```python
from build123d import *

# Parameters (mm, degrees)
SKETCH_1_R              = 8
EXTRUDE_1_DEPTH         = 3
HOLE_WIZARD_M1_21_D     = 1.4
HOLE_WIZARD_M1_21_DEPTH = 9.579397567
HOLE_WIZARD_M1_21_TIP   = 0.420602433
SKETCH_1_3_R            = 18
EXTRUDE_2_DEPTH         = 2
SKETCH_2_W              = 16
SKETCH_2_H              = 7
EXTRUDE_3_DEPTH         = 27
FILLET_1_R              = 6
FILLET_3_R              = 1.5
HOLE_WIZARD_M21_D       = 2.4
HOLE_WIZARD_M21_DEPTH   = 9.278967257
HOLE_WIZARD_M21_TIP     = 0.721032743
HOLE_WIZARD_M1_22_D     = 1.4
HOLE_WIZARD_M1_22_DEPTH = 9.579397567
HOLE_WIZARD_M1_22_TIP   = 0.420602433
FILLET_4_R              = 2


with BuildPart() as part:
    # Sketch 1 → Extrude 1 (new body)
    with BuildSketch(Plane.XY):
        with BuildLine():
            Line((0, 0), (40, 0))
            ThreePointArc((40, 0), (49.772170092, 28), (40, 56))
            Line((40, 56), (0, 56))
            Line((0, 56), (0, 0))
        make_face()
        with Locations((20, 28)):
            Circle(SKETCH_1_R, mode=Mode.SUBTRACT)
    extrude(amount=-EXTRUDE_1_DEPTH)

    # Hole Wizard M1.21
    with Locations(Plane.XY):
        with Locations((20, 41), (31.258330249, 34.5), (31.258330249, 21.5), (20, 15), (8.741669751, 21.5), (8.741669751, 34.5)):
            Hole(HOLE_WIZARD_M1_21_D / 2, depth=HOLE_WIZARD_M1_21_DEPTH)
            with Locations((0, 0, -(HOLE_WIZARD_M1_21_DEPTH + HOLE_WIZARD_M1_21_TIP / 2))):  # 118° drill point
                Cone(0, HOLE_WIZARD_M1_21_D / 2, HOLE_WIZARD_M1_21_TIP, mode=Mode.SUBTRACT)

    # Sketch 1_3 → Extrude 2 (add)
    with BuildSketch(Plane.XY):
        with BuildLine():
            Line((0, 0), (40, 0))
            ThreePointArc((40, 0), (49.772170092, 28), (40, 56))
            Line((40, 56), (0, 56))
            Line((0, 56), (0, 0))
        make_face()
        with Locations((20, 28)):
            Circle(SKETCH_1_3_R, mode=Mode.SUBTRACT)
    extrude(amount=EXTRUDE_2_DEPTH)

    # Sketch 2 → Extrude 3 (add)
    with BuildSketch(Plane.XY.offset(2)):
        with BuildLine():
            Line((40, 0), (12, 0))
            Line((12, 0), (12, 7))
            Line((12, 7), (40, 7))
            Line((40, 7), (40, 49))
            Line((40, 49), (38, 49))
            Line((38, 49), (38, 56))
            Line((38, 56), (40, 56))
            ThreePointArc((40, 56), (49.772170092, 28), (40, 0))
        make_face()
        with Locations((20, 52.5)):
            Rectangle(SKETCH_2_W, SKETCH_2_H)
    extrude(amount=EXTRUDE_3_DEPTH)

    # Fillet 1
    fillet_1_edges = [part.edges().sort_by_distance(p)[0] for p in [
        (40, 56, 13),
        (40, 0, 13),
        (0, 0, -0.5),
        (0, 56, -0.5),
    ]]
    fillet(fillet_1_edges, radius=FILLET_1_R)

    # Fillet 3
    fillet_3_edges = [part.edges().sort_by_distance(p)[0] for p in [
        (12, 7, 15.5),
        (12, 0, 15.5),
        (12, 56, 15.5),
        (12, 49, 15.5),
        (28, 49, 15.5),
        (28, 56, 15.5),
    ]]
    fillet(fillet_3_edges, radius=FILLET_3_R)

    # Hole Wizard M21
    with Locations(Plane.XY.offset(29)):
        with Locations((44, 38), (44, 18)):
            Hole(HOLE_WIZARD_M21_D / 2, depth=HOLE_WIZARD_M21_DEPTH)
            with Locations((0, 0, -(HOLE_WIZARD_M21_DEPTH + HOLE_WIZARD_M21_TIP / 2))):  # 118° drill point
                Cone(0, HOLE_WIZARD_M21_D / 2, HOLE_WIZARD_M21_TIP, mode=Mode.SUBTRACT)

    # Hole Wizard M1.22
    with Locations(Plane.ZY.offset(-12)):
        with Locations((20, 52.240238149), (11, 52.240238149), (20, 3.759761857), (11, 3.759761857)):
            Hole(HOLE_WIZARD_M1_22_D / 2, depth=HOLE_WIZARD_M1_22_DEPTH)
            with Locations((0, 0, -(HOLE_WIZARD_M1_22_DEPTH + HOLE_WIZARD_M1_22_TIP / 2))):  # 118° drill point
                Cone(0, HOLE_WIZARD_M1_22_D / 2, HOLE_WIZARD_M1_22_TIP, mode=Mode.SUBTRACT)

    # Fillet 4
    fillet_4_edges = [part.edges().sort_by_distance(p)[0] for p in [
        (49.772170092, 28, -3),
        (21.487327234, 56, -3),
        (21.487327234, 0, -3),
        (0, 28, -3),
        (1.757359313, 54.242640687, -3),
        (1.757359313, 1.757359313, -3),
        (39.775753154, 0.693980197, -3),
        (39.775753154, 55.306019803, -3),
    ]]
    fillet(fillet_4_edges, radius=FILLET_4_R)


solid = part.part
```
Geometry check sheet. Reference: the model listing, model coordinates, mm. A direction names the side the tool comes from. Round coordinates to 2 decimals unless told otherwise and drop trailing zeros. Order: outer loops, then holes, each group sorted by start corner. A loop starts at its lowest first (then second) coordinate and runs counter-clockwise, first axis right, second up. Notation, with made-up numbers: (29.25, 72.25) - (62.25, 72.25) arc R36 cw to (62.25, 110.25) - close; hole circle Ø11 at (10, 17). An arc over 180 degrees is marked (long way). Use a Markdown table: item, result. Add a question column.
1) Set-up check for faces 5 (the cylindrical face through (42.89, 17.54, 24.3)), 6 (the cylindrical face through (21.27, 55.4, -2.43)), 7 (the flat face through (39, 49, 15)), 8 (the flat face through (0, 28, 0)), 9 (the flat face through (12, 3, 15)): record each of +Z, -Z, +X, -X, +Y, -Y from which the full face is reachable in a straight line by a thin tool's end or side.
2) Section check A-A (z = 21.5). Record the cut outline in (x, y), then the cut area to 3 significant figures.
3) Section check B-B (x = 20). Count the separate pieces of the cut face and the enclosed holes in it, then the cut area to 3 significant figures.
4) Gauge pin test, flat ends, axial feed: P1, Ø1, axis at x = 14.5, y = 32, coming from the +Z side; P2, Ø11, axis at x = 19, y = 21.5, coming from the +Z side; P3, Ø2, axis at y = 53, z = 9, coming from the +X side; P4, Ø2, axis at y = 52, z = 11, coming from the -X side. Record the tip position at first contact, or that the pin passes through.
5) Mould release check, pull along X, two halves, no side actions. Record for faces 1 (the cylindrical face through (1.804, 54.289, 0.479)), 2 (the cylindrical face through (20.152, 40.317, -1.521)), 3 (the cylindrical face through (40.365, 54.95, 14.21)), 4 (the flat face through (20, 49, 15)): released by +X, released by -X, zero draft, split by the parting line, or undercut.
6) Thickness scan on line 1 along Y through (x, z) = (16, 11); line 2 along X through (y, z) = (34, -1); line 3 along Y through (x, z) = (29, 5). Record the ranges inside material, lowest first.
7) Section check C-C (z = 7.5). Record the cut outline in (x, y).
Established:
| question | item | result |
|---|---|---|
| 1 | face 5 | +Z |
| 1 | face 6 | -Z, +X, -X, +Y |
| 1 | face 7 | +Z, -X |
| 1 | face 8 | +Z, -Z, -X, +Y, -Y |
| 1 | face 9 | +Z, -X, +Y, -Y |
| 2 | outline | (12, 1.5) arc R1.5 ccw to (13.5, 0) - (36.97, 0) arc R6 ccw to (41.93, 2.62) arc R45 ccw to (41.93, 53.38) arc R6 ccw to (38, 55.91) - (38, 49) - (40, 49) - (40, 7) - (13.5, 7) arc R1.5 ccw to (12, 5.5) - close; (12, 50.5) arc R1.5 ccw to (13.5, 49) - (26.5, 49) arc R1.5 ccw to (28, 50.5) - (28, 54.5) arc R1.5 ccw to (26.5, 56) - (13.5, 56) arc R1.5 ccw to (12, 54.5) - close; hole circle Ø2.4 at (44, 18); hole circle Ø2.4 at (44, 38) |
| 2 | area | 681 mm2 |
| 3 | separate pieces | 4 |
| 3 | enclosed holes | 4 |
| 3 | area | 522 mm2 |
| 4 | P1 | through |
| 4 | P2 | z = 0 |
| 4 | P3 | x = 42.84 |
| 4 | P4 | x = 12 |
| 5 | face 1 | released by -X |
| 5 | face 2 | undercut |
| 5 | face 3 | released by +X |
| 5 | face 4 | zero draft |
| 6 | line 1 | 0 to 3.06, 4.46 to 7, 49 to 51.54, 52.94 to 56 |
| 6 | line 2 | 0 to 8.25, 9.23 to 14.71, 25.29 to 30.77, 31.75 to 49.37 |
| 6 | line 3 | 0 to 7 |
| 7 | outline | (12, 1.5) arc R1.5 ccw to (13.5, 0) - (36.97, 0) arc R6 ccw to (41.93, 2.62) arc R45 ccw to (41.93, 53.38) arc R6 ccw to (38, 55.91) - (38, 49) - (40, 49) - (40, 7) - (13.5, 7) arc R1.5 ccw to (12, 5.5) - close; (12, 50.5) arc R1.5 ccw to (13.5, 49) - (26.5, 49) arc R1.5 ccw to (28, 50.5) - (28, 54.5) arc R1.5 ccw to (26.5, 56) - (13.5, 56) arc R1.5 ccw to (12, 54.5) - close |
